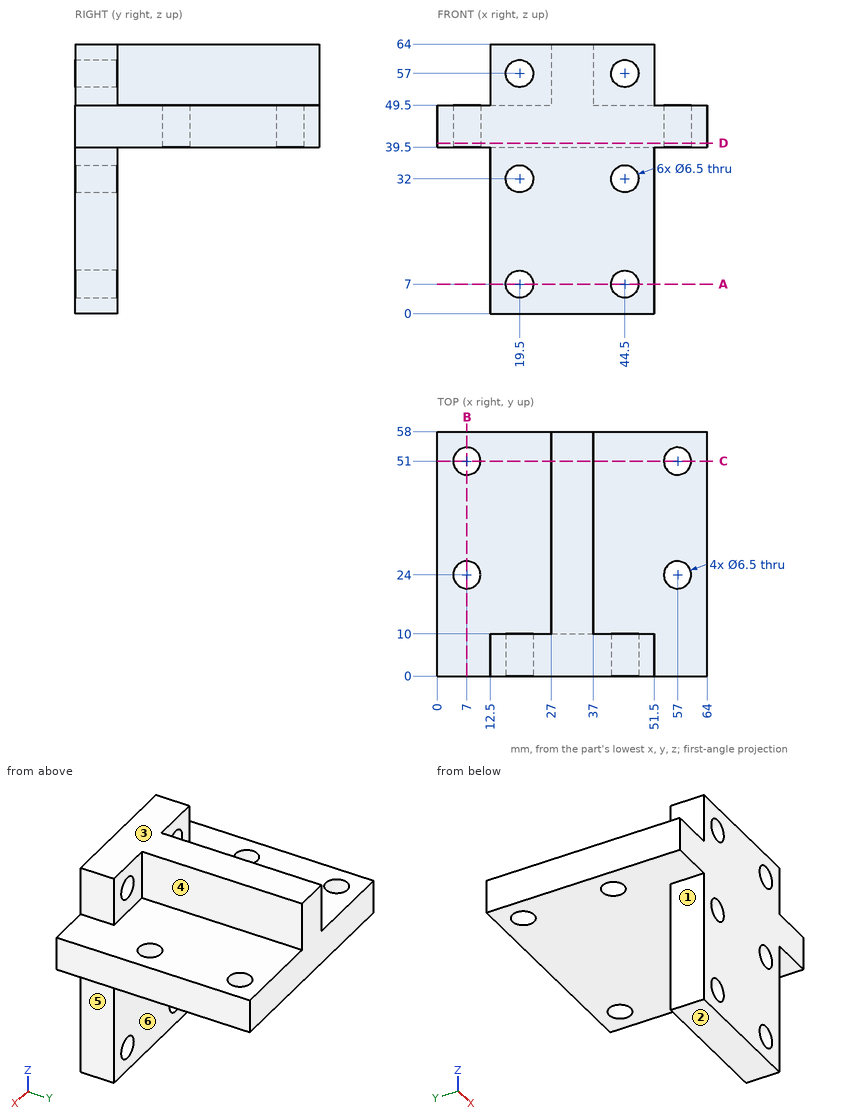
The drawing under review shows one solid part. Ordinate dimensions are in mm from its lowest x, y, z. A direction names the side the tool comes from. Round coordinates to 2 decimals unless told otherwise and drop trailing zeros. Write each loop counter-clockwise with the first axis right and the second up, starting at its lowest first coordinate (ties: lowest second). Pieces come first, ordered by that corner, then holes. Notation, with made-up numbers: (-3.75, -25) -> (7.25, -25) arc R10 cw to (7.25, -19) -> close; hole circle Ø4 at (-30, 71.5). An arc over 180 degrees is marked (long way). One line per question, with ' | ' between items. Start each with the question number.
(1) Add section A-A, the plane z = 7. Write out the cut boundary in (x, y), plus the area to 3 significant figures.
(2) Add section B-B, the plane x = 7. Write out the cut boundary in (y, z), plus the area to 3 significant figures.
(3) Tool access review of the marked faces 4, 5 and 6: name each direction out of +Z, -Z, +X, -X, +Y, -Y from which nothing blocks a thin tool from reaching the whole face with its end or side.
(4) Add section D-D, the plane z = 40.5. Write out the cut boundary in (x, y).
(5) Insertion check: P1, Ø1.5, axis at y = 37.5, z = 54, coming from the -X side; P2, Ø8, axis at x = 40, z = 39.5, coming from the -Y side; P3, Ø4, axis at x = 7, y = 24, coming from the -Z side; P4, Ø4.5, axis at y = 23, z = 55.5, coming from the +X side. Each pin has a flat end and moves straight along its axis. Give the tip position at first contact, or say it passes through.
(6) Add section C-C, the plane y = 51. Write out the cut boundary in (x, z), plus the area to 3 significant figures.
(7) Mouldability with a two-part tool opening along Z and no side actions: class the marked faces 1, 2 and 3 as released by +Z, released by -Z, zero draft, split by the parting line, or undercut.
(8) For line 1 along X through (y, z) = (3.25, 57); line 2 along Z through (x, y) = (45.5, 4); line 3 along X through (y, z) = (7, 31), list the stretches that pass through material, from the lowest coordinate up. Write a range as from..to.
Answer list:
1) outline: (12.5, 0) -> (16.25, 0) -> (16.25, 10) -> (12.5, 10) -> close; (22.75, 0) -> (41.25, 0) -> (41.25, 10) -> (22.75, 10) -> close; (47.75, 0) -> (51.5, 0) -> (51.5, 10) -> (47.75, 10) -> close | area: 260 mm²
2) outline: (0, 39.5) -> (20.75, 39.5) -> (20.75, 49.5) -> (0, 49.5) -> close; (27.25, 39.5) -> (47.75, 39.5) -> (47.75, 49.5) -> (27.25, 49.5) -> close; (54.25, 39.5) -> (58, 39.5) -> (58, 49.5) -> (54.25, 49.5) -> close | area: 450 mm²
3) face 4: +Z, +X, +Y | face 5: -Z, +X, +Y, -Y | face 6: -Z, +X, -X, +Y
4) outline: (0, 0) -> (64, 0) -> (64, 58) -> (0, 58) -> close; hole circle Ø6.5 at (7, 24); hole circle Ø6.5 at (7, 51); hole circle Ø6.5 at (57, 24); hole circle Ø6.5 at (57, 51)
5) P1: x = 27 | P2: y = 0 | P3: through | P4: x = 37
6) outline: (0, 39.5) -> (3.75, 39.5) -> (3.75, 49.5) -> (0, 49.5) -> close; (10.25, 39.5) -> (53.75, 39.5) -> (53.75, 49.5) -> (37, 49.5) -> (37, 64) -> (27, 64) -> (27, 49.5) -> (10.25, 49.5) -> close; (60.25, 39.5) -> (64, 39.5) -> (64, 49.5) -> (60.25, 49.5) -> close | area: 655 mm²
7) face 1: zero draft | face 2: released by -Z | face 3: released by +Z
8) line 1: 12.5..16.25, 22.75..41.25, 47.75..51.5 | line 2: 0..3.91, 10.09..28.91, 35.09..53.91, 60.09..64 | line 3: 12.5..16.41, 22.59..41.41, 47.59..51.5
